Could you check a few things on this model? Use its own coordinates, in mm. Coordinates: 2 decimals unless noted, no trailing zeros. Loops run counter-clockwise (first coordinate to the right, second up) from the corner with the lowest first, then second, coordinate; pieces in that order, holes last. Notation, with made-up numbers: M 41.25,45 L 75.25,45 A9 ccw 75.25,50 Z; hole C 71.25,-39 d2. An arc over 180 degrees is marked long. Write each question's results on one line, items separated by ' | '.
```python
from build123d import *

# Parameters (mm, degrees)
F0_W     = 92.4328938127
F0_H     = 76.2194246054
F1_DEPTH = 50.8
F3_DEPTH = 127
F4_DEPTH = 25.4


with BuildPart() as f1:
    # F0 (on Top) → F1 (new body)
    with BuildSketch(Plane.XY):
        Rectangle(F0_W, F0_H)
    extrude(amount=F1_DEPTH)

    # F2 (on face) → F3 (cut)
    with BuildSketch(Plane.XZ.offset(38.1097123027)):
        Polygon((46.2164469063, 50.8), (-46.2164469063, 50.8), (46.2164469063, 0), align=None)
    extrude(amount=-F3_DEPTH, mode=Mode.SUBTRACT)

    # F4 (add): a face of the model
    f4_faces = [f1.faces().sort_by_distance(p)[0] for p in [
        (-46.2164469063, 0, 25.4),
    ]]
    extrude(f4_faces, amount=F4_DEPTH)


solid = f1.part
```
(1) Imagine slicing it at A-A, the plane y = 3. List the corners of the cut face in (x, z) for me, and give its area (3 significant figures).
Reported:
outline: M -71.62,0 L 46.22,0 L -46.22,50.8 L -71.62,50.8 Z | area: 3,640 mm2
(2) Will these pins go through, and if not, where does the flat tip stop? P1, Ø4, axis at x = 17.5, y = 9.5, coming from the +Z side; P2, Ø3, axis at x = 19.5, y = -10, coming from the +Z side; P3, Ø1.5, axis at x = -30, y = 17, coming from the +Z side.
Reported:
P1: stops at z = 16.88 | P2: stops at z = 15.51 | P3: stops at z = 42.3
(3) Please list where these lines run through material, in increasing order: probe 1 along Z at (x, y) = (29, 4); probe 2 along X at (y, z) = (-5, 24.5); probe 3 along X at (y, z) = (-10.5, 4.5). Write a range as from..to.
Reported:
probe 1: z = 0..9.46 | probe 2: x = -71.62..1.64 | probe 3: x = -71.62..38.03
(4) Imagine slicing it at B-B, the plane x = -35. List the corners of the cut face in (y, z) for me, and give its area (3 significant figures).
Reported:
outline: M -38.11,0 L 38.11,0 L 38.11,44.64 L -38.11,44.64 Z | area: 3,400 mm2
